For this review, take the finished solid that the model builds, in its own axes (mm). A direction names the side the tool comes from. Coordinates: 2 decimals unless noted, no trailing zeros. Write each loop counter-clockwise with the first axis right and the second up, starting at its lowest first coordinate (ties: lowest second). Pieces come first, ordered by that corner, then holes. Notation, with made-up numbers: (59, 80.25) -> (72, 80.25) arc R19 cw to (72, 109.25) -> close; hole circle Ø5 at (12, -33.75). An arc over 180 degrees is marked (long way). One line per item, written item: value. Start each with the question number.
1) Mouldability with a two-part tool opening along X and no side actions: class faces 1 (the cylindrical face through (7.33, 2.31, 9.15)), 2 (the flat face through (-8, -2, 12.7)), 3 (the conical face through (5.06, 1.59, -17.88)) as released by +X, released by -X, zero draft, split by the parting line, or undercut.
2) Add section C-C (z = 1). State the section outline as (x, y) points (3 decimals), and give its area (3 significant figures).
3) For pin 1 Ø2 at (x, z) = (-8, -13) entering from -Y; pin 2 Ø8 at (x, z) = (-4, -4.5) entering from +Y; pin 3 Ø7.5 at (x, y) = (-2, -2.5) entering from +Z, all flat-tipped, find the tip position at first contact; note any pin that passes through.
4) Add section D-D (z = -15). State the section outline as (x, y) points, and give its area (3 significant figures).
5) For probe 1 along Y at (x, z) = (0, 10) (1 decimal); probe 2 along Z at (x, y) = (2.25, 1); probe 3 along Z at (x, y) = (8.5, -4.5), list the stretches that pass through material, from the lowest coordinate up. Write a range as from..to.
6) Machinability: for faces 4 (the flat face through (0, 0, -18)), 5 (the flat face through (-8, -2, 0)), 6 (the flat face through (0, 0, 5.7)), which of the approach directions +Z, -Z, +X, -X, +Y, -Y give a long, thin tool a straight path to every point of the face, cutting with its end or side? Answer none if there is none.
7) Add section A-A (y = 0). State the section outline as (x, z) points (1 decimal).
from build123d import *

# Parameters (mm, degrees)
F0_R     = 11.175
F0_R_2   = 7.6835
F1_DEPTH = 12.7
F2_DEPTH = 18
F3_DEPTH = 5.7
F4_SIZE  = 2.5


# Not quite as in the source:
# - a length typed as a fraction of an inch, garbled in the dataset ("3 / 203.2 mm" for 3/8 in), is restored


with BuildPart() as f1:
    # F0 (on Top) → F1 (new body)
    with BuildSketch(Plane.XY):
        Circle(F0_R)
        Circle(F0_R_2, mode=Mode.SUBTRACT)
    extrude(amount=F1_DEPTH)



with BuildPart() as f2:
    # F0 (on Top) → F2 (new body)
    with BuildSketch(Plane.XY):
        Circle(F0_R_2)
    extrude(amount=-F2_DEPTH)


with BuildPart() as f1_1:
    add(f1.part)

    add(f2.part)  # F3 merges F2
    # F0 (on Top) → F3 (join)
    with BuildSketch(Plane.XY):
        Circle(F0_R_2)
    extrude(amount=F3_DEPTH)

    # F4
    f4_edges = [f1_1.edges().sort_by_distance(p)[0] for p in [
        (-7.6835, 0, -18),
    ]]
    chamfer(f4_edges, length=F4_SIZE)


solid = f1_1.part
Numbers:
1. face 1: undercut
1. face 2: zero draft
1. face 3: split by the parting line
2. outline: circle Ø22.35 at (0, 0)
2. area: 392 mm²
3. pin 1: y = -3.17
3. pin 2: y = 7.68
3. pin 3: z = 5.7
4. outline: circle Ø15.37 at (0, 0)
4. area: 185 mm²
5. probe 1: -11.2..-7.7, 7.7..11.2
5. probe 2: -18..5.7
5. probe 3: 0..12.7
6. face 4: -Z, +X, -X, +Y, -Y
6. face 5: -Z
6. face 6: +Z
7. outline: (-11.2, 0) -> (-7.7, 0) -> (-7.7, -15.5) -> (-5.2, -18) -> (5.2, -18) -> (7.7, -15.5) -> (7.7, 0) -> (11.2, 0) -> (11.2, 12.7) -> (7.7, 12.7) -> (7.7, 5.7) -> (-7.7, 5.7) -> (-7.7, 12.7) -> (-11.2, 12.7) -> close
